Autodesk Inventor part; units mm, degrees
ref_plane "YZ Plane" through (0, 0, 0) normal (1, 0, 0) x (0, 1, 0)
ref_plane "XZ Plane" through (0, 0, 0) normal (0, 1, 0) x (-1, 0, 0)
ref_plane "XY Plane" through (0, 0, 0) normal (0, 0, 1) x (1, 0, 0)
sketch "Sketch1" plane through (0, 0, 0) normal (0, 0, 1) x (1, 0, 0)
  line L0 (-170, -160) -> (170, -160)
  line L1 (170, -160) -> (170, -120)
  line L2 (170, 160) -> (-170, 160)
  line L3 (-170, 160) -> (-170, 120)
  line L4 (-170, -160) -> (170, 160) construction
  line L5 (170, -160) -> (-170, 160) construction
  line L6 (-140, -155) -> (140, -155) construction
  line L7 (140, -155) -> (140, 155) construction
  line L8 (140, 155) -> (-140, 155) construction
  line L9 (-140, 155) -> (-140, -155) construction
  line L10 (-140, -155) -> (140, 155) construction
  line L11 (140, -155) -> (-140, 155) construction
  line L12 (-150, -150) -> (150, -150) construction
  line L13 (150, -150) -> (150, 150) construction
  line L14 (150, 150) -> (-150, 150) construction
  line L15 (-150, 150) -> (-150, -150) construction
  line L16 (-150, -150) -> (150, 150) construction
  line L17 (150, -150) -> (-150, 150) construction
  line L18 (170, 120) -> (150, 120)
  line L19 (150, 120) -> (150, 98)
  line L20 (150, 98) -> (170, 98)
  line L21 (170, 98) -> (170, 120) construction
  line L22 (0, -160) -> (0, 160) construction
  line L23 (-170, 0) -> (170, 0) construction
  line L24 (-170, 120) -> (-150, 120)
  line L25 (-150, 120) -> (-150, 98)
  line L26 (-150, 98) -> (-170, 98)
  line L27 (-170, 98) -> (-170, 120) construction
  line L28 (170, -120) -> (150, -120)
  line L29 (150, -120) -> (150, -98)
  line L30 (150, -98) -> (170, -98)
  line L31 (170, -98) -> (170, -120) construction
  line L32 (-170, -120) -> (-150, -120)
  line L33 (-150, -98) -> (-170, -98)
  line L34 (-170, -98) -> (-170, -120) construction
  line L35 (-150, -120) -> (-150, -98)
  line L36 (-170, 98) -> (-170, -98)
  line L37 (-170, -120) -> (-170, -160)
  line L38 (-170, -98) -> (-170, -120)
  line L39 (170, -120) -> (170, -98)
  line L40 (170, -98) -> (170, 98)
  line L41 (170, 98) -> (170, 120)
  line L42 (170, 120) -> (170, 160)
  line L43 (-170, 120) -> (-170, 98) construction
  line L44 (170, 12) -> (150, 12)
  line L45 (150, 12) -> (150, -12)
  line L46 (150, -12) -> (170, -12)
  line L47 (170, -12) -> (170, 12)
  point P0 (0, 0)
  point P1 (0, 0)
  dimension "d0" = 340
  dimension "d1" = 320
  dimension "d4" = 280
  dimension "d5" = 310
  dimension "d13" = 300
  dimension "d14" = 300
  dimension "d15" = 22
  dimension "d16" = 30
  dimension "d27" = 24
extrude "Extrusion1" add sketch "Sketch1" along normal blind 4 contours L37 L32 L35 L33 L36 L26 L25 L24 L3 L2 L42 L18 L19 L20 L40 L44 L45 L46 L30 L29 L28 L1 L0
hole "Hole1" at (-140, 155, 0) at (-140, -155, 0) at (140, -155, 0) at (140, 155, 0) at (0, 0, 0) direction (0, 0, 1) diameter 3.2 end through all
sketch "Szkic2" plane through (0, 0, 4) normal (0, 0, 1) x (1, 0, 0)
  point P0 (-150, 98)
  point P1 (-150, 120)
  point P2 (-150, -120)
  point P3 (-150, -98)
  point P4 (150, -120)
  point P5 (150, -98)
  point P6 (150, 98)
  point P7 (150, 120)
  point P8 (150, 12)
  point P9 (150, -12)
hole "Otwór2" at (-150, 98, 4) at (-150, 120, 4) at (-150, -120, 4) at (-150, -98, 4) at (150, -120, 4) at (150, -98, 4) at (150, 98, 4) at (150, -12, 4) at (150, 12, 4) at (150, 120, 4) direction (0, 0, -1) diameter 1 end through all
chamfer "Faza1" distance 5 angle 45 4 edges at (-170, -160, 2) (170, -160, 2) (170, 160, 2) (-170, 160, 2)
chamfer "Faza2" distance 2 angle 45 10 edges at (170, -120, 2) (170, -98, 2) (170, -12, 2) (170, 12, 2) (170, 98, 2) (170, 120, 2) (-170, -120, 2) (-170, -98, 2) (-170, 120, 2) (-170, 98, 2)
properties part number "stolik"
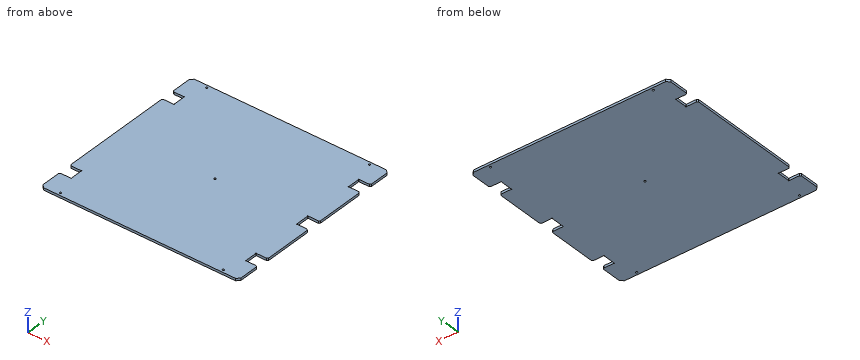
CAD build for the part. Positions are in the model's coordinates, mm. Round coordinates to 2 decimals unless told otherwise and drop trailing zeros. Write item = value, one per line. Start each with the question number.
Q1. Band-saw the part on A-A (z = 1.8). Count the separate pieces of the cut face and the enclosed holes in it, then the cut area to 3 significant figures.
Q2. Drop flat-ended pins along their axis: pin 1 (3 mm diameter, centred on x = 140, y = -155, fed in from -Z); pin 2 (1.2 mm diameter, centred on y = 109.5, z = 2.5, fed in from -X). Give the stop position or say it passes through.
Q3. Probe L1, parallel to Y at x = 140, z = 0.9; L2, parallel to X at y = 0, z = 2; L3, parallel to Y at x = 0.5, z = 2.6. List the from-to ranges inside material, lowest first. Write a range as from..to.
Answers below:
q1.separate_pieces = 1
q1.enclosed_holes = 5
q1.area = 106,000 mm2
q2.pin_1 = through
q2.pin_2 = -150
q3.L1 = -160..-156.6, -153.4..153.4, 156.6..160
q3.L2 = -170..-1.6, 1.6..150
q3.L3 = -160..-1.52, 1.52..160
